from build123d import *

# Parameters (mm, degrees)
SKETCH_1_R      = 2.6
SKETCH_1_R_2    = 7.5
EXTRUDE_1_DEPTH = 20


with BuildPart() as part:
    # 草图1 → 凸台-拉伸1 (new body)
    with BuildSketch(Plane.XY):
        with BuildLine():
            Line((-90.182622834, -3.687217222), (-165.784023014, -69.142761608))
            ThreePointArc((-165.784023014, -69.142761608), (-167.305901383, -90.301303292), (-146.147359698, -91.823181662))
            Line((-146.147359698, -91.823181662), (-99.206677775, -51.182031077))
            ThreePointArc((-99.206677775, -51.182031077), (-70.96175344, -30.746669364), (-39.59736965, -15.526446352))
            Line((-39.59736965, -15.526446352), (172.570702611, 65.433053226))
            Line((172.570702611, 65.433053226), (161.875435514, 93.461810989))
            Line((161.875435514, 93.461810989), (-85.711924724, -1.013048368))
            ThreePointArc((-85.711924724, -1.013048368), (-88.064253508, -2.154565094), (-90.182622834, -3.687217222))
        make_face()
        with Locations((157.880149808, 75.882343075)):
            Circle(SKETCH_1_R, mode=Mode.SUBTRACT)
        with Locations((83.136795774, 47.361630817)):
            Circle(SKETCH_1_R_2, mode=Mode.SUBTRACT)
    extrude(amount=EXTRUDE_1_DEPTH)


solid = part.part
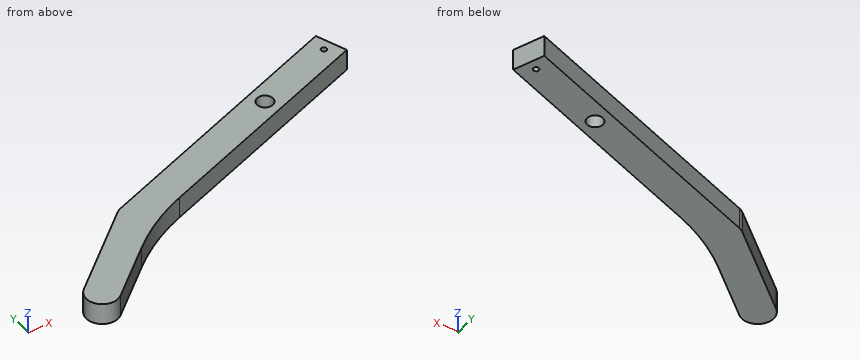
Geometry: final body of the model. Coordinates: model frame, mm. Give positions to 0.01 mm unless a question says otherwise; leave off trailing zeros. Write each loop counter-clockwise with the first axis right and the second up, starting at its lowest first coordinate (ties: lowest second). Pieces come first, ordered by that corner, then holes.
(1) Cut plane C-C, the plane x = 19.5. Return loops of the section in (y, z).
(2) Ray query, line 1 (Y direction, x = 156.5, z = 1.5); line 2 (X direction, y = -86, z = 1.75); line 3 (Y direction, x = 102.5, z = 13.5). Return the intervals inside material, ascending.
(3) Cut plane D-D, the plane y = 16. Return loops of the section in (x, z), then the cut area to 3 significant figures.
(4) Cut plane A-A, the plane z = 6.5. Return loops of the section in (x, y), then the cut area to 3 significant figures.
(5) First-contact query: P1, Ø1, axis at x = 34.5, y = 21.5, coming from the -Z side; P2, Ø1, axis at x = 62, z = 5.5, coming from the +Y side; P3, Ø10, axis at x = 31, z = 16, coming from the -Y side; P4, Ø5, axis at y = -48, z = 7.5, coming from the -X side. Flat tips, straight axial feed; report the tip coordinate or a pass-through.
(6) Cut plane B-B, the plane y = 44. Return loops of the section in (x, z), then the cut area to 3 significant figures.
Values follow:
1. outline: (7.02, 0) - (39.13, 0) - (39.13, 20) - (7.02, 20) - close
2. line 1: y = 59.3 to 73.68, 78.09 to 91.41
2. line 2: x = -169.91 to -139.42
2. line 3: y = 38.7 to 70.81
3. outline: (-41.13, 0) - (43.02, 0) - (43.02, 20) - (-41.13, 20) - close
3. area: 1,680 mm2
4. outline: (-165.78, -69.14) arc R15 ccw to (-146.15, -91.82) - (-99.21, -51.18) arc R200 cw to (-39.6, -15.53) - (172.57, 65.43) - (161.88, 93.46) - (-85.71, -1.01) arc R15 ccw to (-90.18, -3.69) - close; hole circle Ø15 at (83.14, 47.36); hole circle Ø5.2 at (157.88, 75.88)
4. area: 11,200 mm2
5. P1: stops at z = 0
5. P2: stops at y = 55.54
5. P3: stops at y = 9.5
5. P4: stops at x = -144.25
6. outline: (32.25, 0) - (76.43, 0) - (76.43, 20) - (32.25, 20) - close; (89.84, 0) - (116.4, 0) - (116.4, 20) - (89.84, 20) - close
6. area: 1,410 mm2
